Could you check a few things on this drawing? It's one solid part, dimensions in mm from its lowest x, y, z. A direction names the side the tool comes from. Give positions to 0.01 mm unless a question says otherwise; leave off trailing zeros. Order: outer loops, then holes, each group sorted by start corner. A loop starts at its lowest first (then second) coordinate and runs counter-clockwise, first axis right, second up.
Item 1: I want a section at D-D, the plane z = 14. Write out the boundary of the cut face in (x, y).
Item 2: If we mould it in two halves opening along Z, with no side actions, what happens to the marked faces 1, 2, 3 and 4? For each: +Z half, -Z half, draft (parallel to the pull), parting line (faces both ways), or undercut.
Item 3: Which directions (+Z, -Z, +X, -X, +Y, -Y) give clear straight access to the entire face, cutting with the end or side of a thin tool? Please do the marked faces 5 and 6.
Item 4: I'm going to push flat-ended pins straight in: pin 1 Ø6 at (y, z) = (19, 10) entering from +X; pin 2 Ø3.5 at (x, y) = (1.5, 10) entering from +Z; pin 3 Ø2 at (y, z) = (8.5, 6) entering from +X; pin 4 Ø4 at (x, z) = (10, 11) entering from -Y. Where does each tip first touch, or does it pass through?
Item 5: If I drill on line 1 along Z through (x, y) = (10.25, 3.5); line 2 along X through (y, z) = (9.25, 5.75); line 3 along X through (y, z) = (18.5, 11.25), over which ranges is the centre line in solid material (lowest first)?
Item 6: I want a section at C-C, the plane x = 14. Write out the boundary of the cut face in (y, z).
Item 7: I want a section at A-A, the plane y = 5. Write out the boundary of the cut face in (x, z).
Item 8: I want a section at B-B, the plane y = 16.75. Write out the boundary of the cut face in (x, z), then the cut area to 3 significant figures.
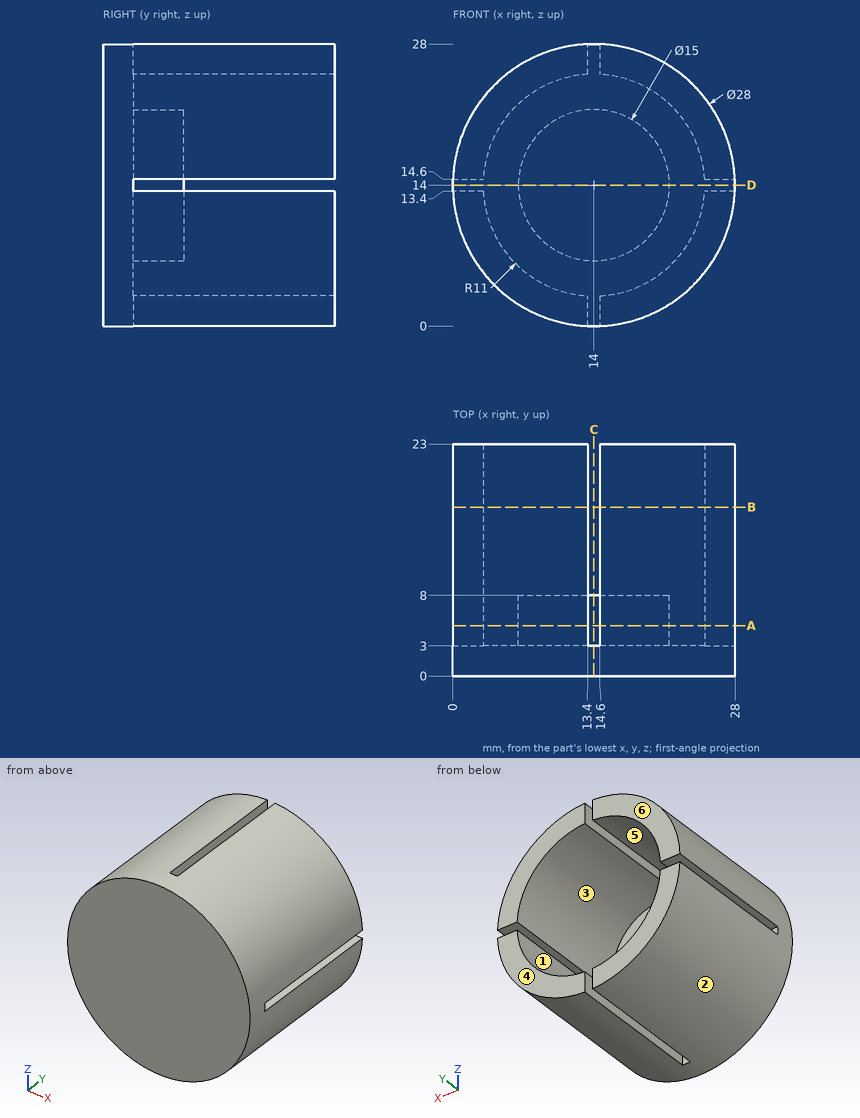
Results list:
1. outline: (0, 0) - (28, 0) - (28, 3) - (21.5, 3) - (21.5, 8) - (6.5, 8) - (6.5, 3) - (0, 3) - close
2. face 1: undercut
2. face 2: parting line
2. face 3: undercut
2. face 4: draft
3. face 5: +Y
3. face 6: +Z, -Z, +X, -X, +Y
4. pin 1: stops at x = 27.96
4. pin 2: stops at z = 22.97
4. pin 3: stops at x = 26.12
4. pin 4: stops at y = 0
5. line 1: z = 0.51 to 3.66, 7.5 to 20.5, 24.34 to 27.49
5. line 2: x = 2.69 to 6.72, 21.28 to 25.31
5. line 3: x = 0.27 to 3.35, 24.65 to 27.73
6. outline: (0, 0) - (3, 0) - (3, 6.5) - (8, 6.5) - (8, 21.5) - (3, 21.5) - (3, 28) - (0, 28) - close
7. outline: (0.01, 13.4) arc R14 ccw to (13.4, 0.01) - (13.4, 3.02) arc R11 cw to (3.02, 13.4) - close; (0.01, 14.6) - (3.02, 14.6) arc R11 cw to (13.4, 24.98) - (13.4, 27.99) arc R14 ccw to start; circle Ø15 at (14, 14); (14.6, 0.01) arc R14 ccw to (27.99, 13.4) - (24.98, 13.4) arc R11 cw to (14.6, 3.02) - close; (14.6, 24.98) arc R11 cw to (24.98, 14.6) - (27.99, 14.6) arc R14 ccw to (14.6, 27.99) - close
8. outline: (0.01, 13.4) arc R14 ccw to (13.4, 0.01) - (13.4, 3.02) arc R11 cw to (3.02, 13.4) - close; (0.01, 14.6) - (3.02, 14.6) arc R11 cw to (13.4, 24.98) - (13.4, 27.99) arc R14 ccw to start; (14.6, 0.01) arc R14 ccw to (27.99, 13.4) - (24.98, 13.4) arc R11 cw to (14.6, 3.02) - close; (14.6, 24.98) arc R11 cw to (24.98, 14.6) - (27.99, 14.6) arc R14 ccw to (14.6, 27.99) - close
8. area: 221 mm2
